```python
from build123d import *

# Parameters (mm, degrees)
SKETCH1_W           = 14
SKETCH1_H           = 34
BOSS_EXTRUDE1_DEPTH = 3
SKETCH2_W           = 7
SKETCH2_H           = 34
BOSS_EXTRUDE2_DEPTH = 5
SKETCH3_R           = 2
CUT_EXTRUDE1_DEPTH  = 5


with BuildPart() as part:
    # Sketch1 → Boss-Extrude1 (new body)
    with BuildSketch(Plane(origin=(0, 0, 0), x_dir=(1, 0, 0), z_dir=(0, 1, 0))):
        Rectangle(SKETCH1_W, SKETCH1_H)
    extrude(amount=BOSS_EXTRUDE1_DEPTH)

    # Sketch2 → Boss-Extrude2 (add)
    with BuildSketch(Plane(origin=(0, 3, 0), x_dir=(1, 0, 0), z_dir=(0, 1, 0))):
        with Locations((-3.5, 0)):
            Rectangle(SKETCH2_W, SKETCH2_H)
    extrude(amount=BOSS_EXTRUDE2_DEPTH)

    # Sketch3 → Cut-Extrude1 (cut)
    with BuildSketch(Plane(origin=(0, 3, 0), x_dir=(1, 0, 0), z_dir=(0, 1, 0))):
        with Locations((3.263282708, -12.5)):
            Circle(SKETCH3_R)
        with Locations((3.263282708, 12.5)):
            Circle(SKETCH3_R)
    extrude(amount=-CUT_EXTRUDE1_DEPTH, mode=Mode.SUBTRACT)


solid = part.part
```
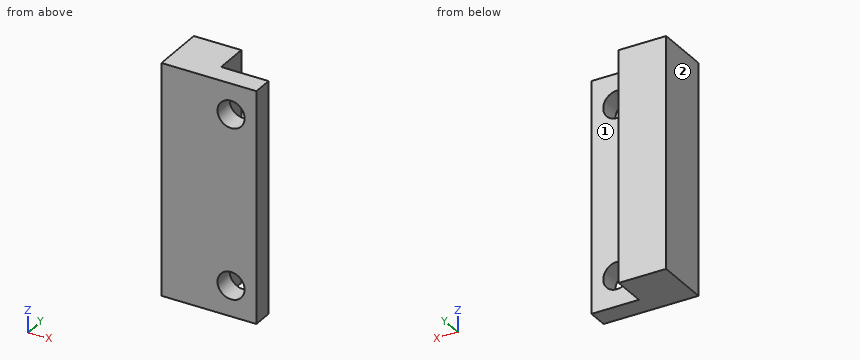
Verification items for the finished model (mm, model axes). Face numbers are marked on the shaded views. A direction names the side the tool comes from. Round coordinates to 2 decimals unless told otherwise and drop trailing zeros. Write each loop counter-clockwise with the first axis right and the second up, starting at its lowest first coordinate (ties: lowest second). Pieces come first, ordered by that corner, then holes. Notation, with made-up numbers: (-32, -14.75) - (-26, -14.75) arc R19 ccw to (-26, 1.25) - close; hole circle Ø4 at (70.5, 29). An arc over 180 degrees is marked (long way). Answer as a JSON object with one key per item and string values. Group by question number.
Q1. Thickness scan on line 1 (X direction, y = 1, z = -12.5); line 2 (Z direction, x = 2.75, y = 2.25); line 3 (Z direction, x = 1.75, y = 2.25). Record the ranges inside material, lowest first.
Q2. Section check A-A, the plane z = 12.5. Enter the section's corners in (x, y).
Q3. Go/stop test with flat-tipped pins: pin 1 Ø2.5 at (x, z) = (3.26, -12.5) entering from -Y; pin 2 Ø3.5 at (x, z) = (3, -1.5) entering from +Y. Record where each tip stops, or that it passes through.
Q4. Tool access check on the marked faces 1 and 2. Record the directions out of +Z, -Z, +X, -X, +Y, -Y that give a thin tool (end or side, any length) a straight path to the whole face; none if there is none.
Q5. Section check D-D, the plane z = 2. Enter the section's corners in (x, y), plus the area to 3 significant figures.
Q6. Section check B-B, the plane x = 4.75. Enter the section's corners in (y, z), plus the area to 3 significant figures.
Q7. Section check C-C, the plane y = 1.5. Enter the section's corners in (x, z).
Found:
{
 "1": {"line 1": "x = -7 to 1.26, 5.26 to 7", "line 2": "z = -17 to -14.43, -10.57 to 10.57, 14.43 to 17", "line 3": "z = -17 to -13.81, -11.19 to 11.19, 13.81 to 17"},
 "2": {"outline": "(-7, 0) - (1.26, 0) - (1.26, 3) - (0, 3) - (0, 8) - (-7, 8) - close; (5.26, 0) - (7, 0) - (7, 3) - (5.26, 3) - close"},
 "3": {"pin 1": "passes through", "pin 2": "stops at y = 3"},
 "4": {"face 1": "+Z, -Z, +X, +Y", "face 2": "+Z, -Z, -X, +Y, -Y"},
 "5": {"outline": "(-7, 0) - (7, 0) - (7, 3) - (0, 3) - (0, 8) - (-7, 8) - close", "area": "77.0 mm^2"},
 "6": {"outline": "(0, -17) - (3, -17) - (3, -13.84) - (0, -13.84) - close; (0, -11.16) - (3, -11.16) - (3, 11.16) - (0, 11.16) - close; (0, 13.84) - (3, 13.84) - (3, 17) - (0, 17) - close", "area": "85.9 mm^2"},
 "7": {"outline": "(-7, -17) - (7, -17) - (7, 17) - (-7, 17) - close; hole circle Ø4 at (3.26, -12.5); hole circle Ø4 at (3.26, 12.5)"}
}
